The figure shows three views and two pictorial views of one solid part (mm, origin at its lowest corner). Answer the questions. Give positions to 0.01 mm unless a question says otherwise; leave off trailing zeros. Write each loop counter-clockwise with the first axis right and the second up, starting at its lowest first coordinate (ties: lowest second). Pieces come first, ordered by that corner, then holes. Notation, with made-up numbers: (61.5, 12.5) -> (77.5, 12.5) arc R9 ccw to (77.5, 28.5) -> close; hole circle Ø1 at (6, 38). An arc over 180 degrees is marked (long way). Answer as CSV lines item,"result". Start each with the question number.
1. The part is cut by section B-B, the plane y = 2.55. Determine the outline of the cut face in (x, z), and give its area (3 significant figures).
2. The part is cut by section C-C, the plane z = 12.25. Determine the outline of the cut face in (x, y), and give its area (3 significant figures).
3. Given pin 1 (4 mm diameter, centred on x = 4, z = 10, fed in from +Y), flat-ended and moving along its own axis, determine where the tip first touches the part or whether it passes through.
4. Find the intervals of material crossed by line 1 (Z direction, x = 11.5, y = 2.3); line 2 (Y direction, x = 3, z = 2.5), in increasing order.
5. For a pull along X with two mould halves and no side action, classify the marked faces 1, 2 and 3 as pulls with the +X half, pulls with the -X half, needs draft (parallel to the pull), parting line crosses it, or undercut.
6. The part is cut by section A-A, the plane x = 14.25. Determine the outline of the cut face in (y, z).
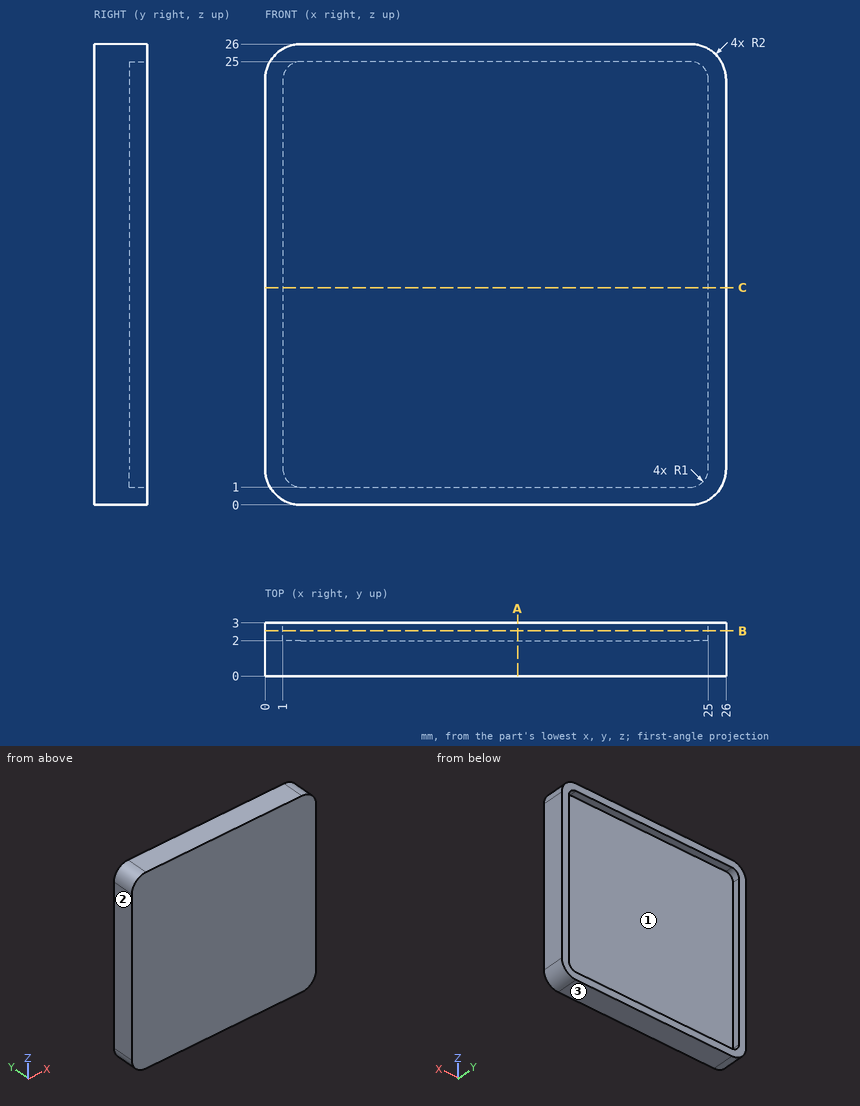
Results found:
1,outline,"(0, 2) arc R2 ccw to (2, 0) -> (24, 0) arc R2 ccw to (26, 2) -> (26, 24) arc R2 ccw to (24, 26) -> (2, 26) arc R2 ccw to (0, 24) -> close; hole (1, 2) arc R1 ccw to (2, 1) -> (24, 1) arc R1 ccw to (25, 2) -> (25, 24) arc R1 ccw to (24, 25) -> (2, 25) arc R1 ccw to (1, 24) -> close"
1,area,"97.4 mm²"
2,outline,"(0, 0) -> (26, 0) -> (26, 3) -> (25, 3) -> (25, 2) -> (1, 2) -> (1, 3) -> (0, 3) -> close"
2,area,"54.0 mm²"
3,pin 1,"stops at y = 2"
4,line 1,"z = 0 to 1, 25 to 26"
4,line 2,"y = 0 to 2"
5,face 1,"undercut"
5,face 2,"pulls with the -X half"
5,face 3,"needs draft"
6,outline,"(0, 0) -> (3, 0) -> (3, 1) -> (2, 1) -> (2, 25) -> (3, 25) -> (3, 26) -> (0, 26) -> close"
